Verification items for the finished model (mm, model axes). Coordinates: 2 decimals unless noted, no trailing zeros. Loops run counter-clockwise (first coordinate to the right, second up) from the corner with the lowest first, then second, coordinate; pieces in that order, holes last. Notation, with made-up numbers: (72, 53.5) -> (98, 53.5) arc R18 cw to (98, 71.5) -> close; hole circle Ø7 at (-9.5, -16). An arc over 180 degrees is marked (long way). Use CSV: the item, a comma, the result in double quotes. Start each with the question number.
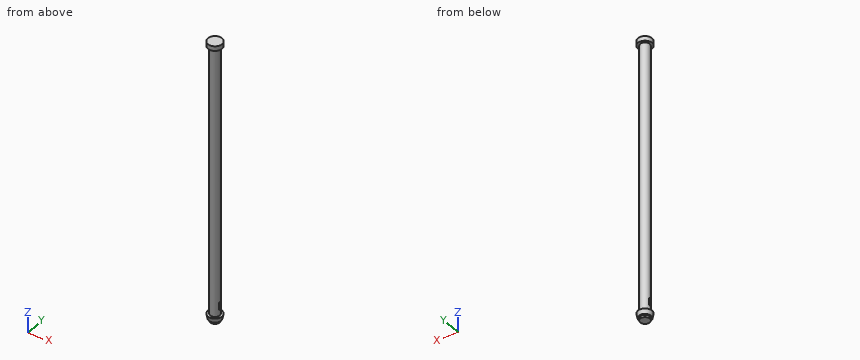
```python
from build123d import *

# Parameters (mm, degrees)
SKETCH1_R               = 10
BOSS_EXTRUDE1_DEPTH     = 590
SKETCH2_R               = 15
BOSS_EXTRUDE2_DEPTH     = 10
SKETCH3_R               = 15
BOSS_EXTRUDE3_DEPTH     = 10
BOSS_EXTRUDE3_TAPER     = 12
BODY_MOVE_COPY1_ANGLE   = 90
SKETCH4_W               = 20
SKETCH4_H               = 15.783753313
CUT_EXTRUDE1_DEPTH      = 2
CUT_EXTRUDE1_DEPTH_BACK = 2


with BuildPart() as part:
    # Sketch1 → Boss-Extrude1 (new body)
    with BuildSketch(Plane(origin=(0, 0, 0), x_dir=(1, 0, 0), z_dir=(0, 1, 0))):
        Circle(SKETCH1_R)
    extrude(amount=BOSS_EXTRUDE1_DEPTH)

    # Sketch2 → Boss-Extrude2 (add)
    with BuildSketch(Plane(origin=(0, 590, 0), x_dir=(1, 0, 0), z_dir=(0, 1, 0))):
        Circle(SKETCH2_R)
    extrude(amount=BOSS_EXTRUDE2_DEPTH)

    # Sketch3 → Boss-Extrude3 (add)
    with BuildSketch(Plane(origin=(0, 15, 0), x_dir=(-1, 0, 0), z_dir=(0, -1, 0))):
        Circle(SKETCH3_R)
    extrude(amount=BOSS_EXTRUDE3_DEPTH, taper=BOSS_EXTRUDE3_TAPER)


with BuildPart() as part_1:
    # Body-Move_Copy1: moved
    add(part.part.rotate(Axis((0, 0, 0), (1, 0, 0)), BODY_MOVE_COPY1_ANGLE))

    # Sketch4 → Cut-Extrude1 (cut, two sides)
    with BuildSketch(Plane(origin=(0, 0, 0), x_dir=(1, 0, 0), z_dir=(0, 1, 0))) as cut_extrude1_sk:
        with Locations((0, -35.976721821)):
            Rectangle(SKETCH4_W, SKETCH4_H)
    extrude(amount=CUT_EXTRUDE1_DEPTH, mode=Mode.SUBTRACT)
    extrude(cut_extrude1_sk.sketch, amount=-CUT_EXTRUDE1_DEPTH_BACK, mode=Mode.SUBTRACT)


solid = part_1.part
```
1. Cross-section at A-A, the plane x = 0. Record the boundary of the cut face in (y, z).
2. Depth check by flat-ended pin: pin 1 (17.5 mm diameter, centred on x = 0.5, z = 37, fed in from +Y); pin 2 (6 mm diameter, centred on x = 11, y = -7, fed in from -Z); pin 3 (5 mm diameter, centred on y = -3, z = 242, fed in from -X). Enter the tip coordinate at first touch or a pass-through.
3. Cross-section at B-B, the plane z = 193. Record the boundary of the cut face in (x, y).
4. Scan lines: line 1 (Z direction, x = -12, y = -1); line 2 (Z direction, x = 9.5, y = -0.5); line 3 (Y direction, x = -1, z = 238). Record each from-to range of solid material in increasing order.
Solution:
1,outline,"(-15, 15) -> (-12.87, 5) -> (-10, 5) -> (-10, 0) -> (10, 0) -> (10, 5) -> (12.87, 5) -> (15, 15) -> (10, 15) -> (10, 590) -> (15, 590) -> (15, 600) -> (-15, 600) -> (-15, 590) -> (-10, 590) -> (-10, 15) -> close; hole (-2, 28.08) -> (2, 28.08) -> (2, 43.87) -> (-2, 43.87) -> close"
2,pin 1,"stops at y = 10"
2,pin 2,"stops at z = 5"
2,pin 3,"stops at x = -9.99"
3,outline,"circle Ø20 at (0, 0)"
4,line 1,"z = 5 to 15, 590 to 600"
4,line 2,"z = 0 to 28.08, 43.87 to 600"
4,line 3,"y = -9.95 to 9.95"
